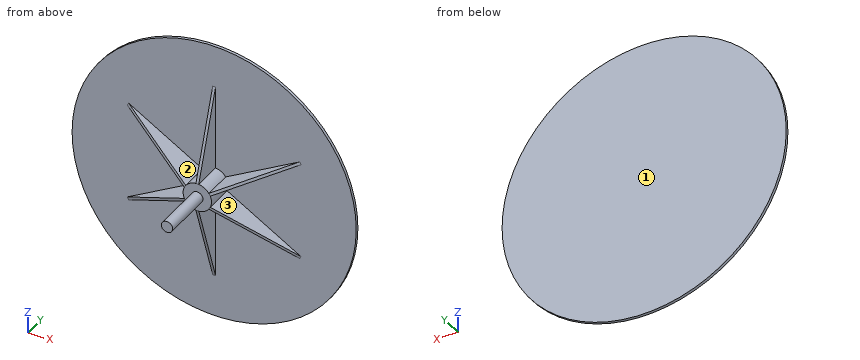
from build123d import *

# Parameters (mm, degrees)
F0_R     = 250
F1_DEPTH = 5
F2_R     = 25
F3_DEPTH = 50
F4_R     = 10
F5_DEPTH = 90
F7_DEPTH = 2.5
F8_COUNT = 6


with BuildPart() as f1:
    # F0 (on Front) → F1 (new body)
    with BuildSketch(Plane.XZ):
        Circle(F0_R)
    extrude(amount=F1_DEPTH)

    # F2 (on face) → F3 (join)
    with BuildSketch(Plane.XZ.offset(5)):
        Circle(F2_R)
    extrude(amount=F3_DEPTH)

    # F4 (on face) → F5 (join)
    with BuildSketch(Plane.XZ.offset(55)):
        Circle(F4_R)
    extrude(amount=F5_DEPTH)

    # F6 (on Right) → F7 (join, symmetric)
    with BuildSketch(Plane.YZ):
        Polygon((-5, 175.0694811344), (-55, 24.9402336776), (-5, 24.9402336776), align=None)
    extrude(amount=F7_DEPTH, both=True)

    # F8: F1 ×6 about axis
    f8_axis = Axis((0, -55, 0), (0, -1, 0))


with BuildPart() as f1_1:
    add(f1.part)
    for i in range(1, F8_COUNT):
        add(f1.part.rotate(f8_axis, i * 360 / F8_COUNT))


solid = f1_1.part
Here's how the part is built. I have some questions about the finished solid (model axes, mm). Face numbers are marked on the shaded views. Round coordinates to 2 decimals unless told otherwise and drop trailing zeros. Write each loop counter-clockwise with the first axis right and the second up, starting at its lowest first coordinate (ties: lowest second). Pieces come first, ordered by that corner, then holes.
1. Suppose I cut it at B-B (x = -90). List the corners of the cut face in (y, z) for me.
2. I need wall thicknesses on L1, parallel to Y at x = 7, z = 185.5; L2, parallel to Z at x = 51.5, y = -18. Which ranges of each line are inside material? Lowest first, please.
3. Suppose I cut it at D-D (z = -64). List the corners of the cut face in (x, y) for me.
4. If we mould it in two halves opening along X, with no side actions, what happens to the marked faces 1, 2 and 3? For each: released by +X, released by -X, zero draft, split by the parting line, or undercut.
5. Suppose I cut it at C-C (y = -134.5). List the corners of the cut face in (x, z) for me, and give its area (3 significant figures).
6. Will these pins go through, and if not, where does the flat tip stop? pin 1 Ø1 at (x, z) = (-189, 161.5) entering from -Y; pin 2 Ø25 at (y, z) = (-36, -113.5) entering from -X; pin 3 Ø8 at (x, y) = (53.5, -18.5) entering from -Z.
7. Suppose I cut it at A-A (z = 0). List the corners of the cut face in (x, y) for me, and give its area (3 significant figures).
Answer sheet:
1. outline: (-29.18, -49.07) - (-28.21, -54.85) - (-5, -54.85) - (-5, -233.24) - (0, -233.24) - (0, 233.24) - (-5, 233.24) - (-5, 54.85) - (-28.21, 54.85) - (-29.18, 49.07) - (-5, 49.07) - (-5, -49.07) - close
2. L1: y = -5 to 0
2. L2: z = -32.62 to -26.85, 26.85 to 32.62
3. outline: (-241.67, -5) - (-115.85, -5) - (-115.85, -19.23) - (-105.85, -22.12) - (-105.85, -5) - (-2.5, -5) - (-2.5, -41.99) - (2.5, -41.99) - (2.5, -5) - (105.85, -5) - (105.85, -22.12) - (115.85, -19.23) - (115.85, -5) - (241.67, -5) - (241.67, 0) - (-241.67, 0) - close
4. face 1: zero draft
4. face 2: undercut
4. face 3: released by +X
5. outline: circle Ø20 at (0, 0)
5. area: 314 mm2
6. pin 1: stops at y = -5
6. pin 2: stops at x = -2.5
6. pin 3: stops at z = -36.08
7. outline: (-250, -5) - (-25, -5) - (-25, -55) - (-10, -55) - (-10, -145) - (10, -145) - (10, -55) - (25, -55) - (25, -5) - (250, -5) - (250, 0) - (-250, 0) - close
7. area: 6,800 mm2
